Source: CAD feature listing. Evaluate the final solid. Frame: model axes, mm. A direction names the side the tool comes from. Coordinates: 2 decimals unless noted, no trailing zeros. Order: outer loops, then holes, each group sorted by start corner. A loop starts at its lowest first (then second) coordinate and runs counter-clockwise, first axis right, second up. Notation, with made-up numbers: (-37.5, -12.75) -> (-22.5, -12.75) arc R12 ccw to (-22.5, 2.25) -> close; hole circle Ø6 at (-4, 84.5). An arc over 180 degrees is marked (long way). Put each result on its own line as item: value.
from build123d import *

# Parameters (mm, degrees)
F1_DEPTH = 1200
F2_R     = 2


# Not quite as in the source:
# - a feature names something its author has since deleted; it is built from what else it names


with BuildPart() as f1:
    # F0 (on Right) → F1 (new body)
    with BuildSketch(Plane.YZ):
        Polygon((-19.8378913403, 177.8021101952), (-19.8378913403, 154.8021101952), (-17.8378913403, 154.8021101952), (-17.8378913403, 179.8021101952), (-57.8378913403, 179.8021101952), (-57.8378913403, 79.8021101952), (-29.8378913403, 79.8021101952), (-29.8378913403, 53.8021101952), (-27.8378913403, 53.8021101952), (-27.8378913403, 81.8021101952), (-55.8378913403, 81.8021101952), (-55.8378913403, 177.8021101952), align=None)
    extrude(amount=F1_DEPTH)

    # F2
    f2_edges = [f1.edges().sort_by_distance(p)[0] for p in [
        (600, -57.837891, 179.80211),
        (600, -17.837891, 179.80211),
        (600, -57.837891, 79.80211),
        (600, -27.837891, 81.80211),
        (600, -55.837891, 81.80211),
        (600, -29.837891, 79.80211),
        (600, -19.837891, 177.80211),
        (600, -55.837891, 177.80211),
    ]]
    fillet(f2_edges, radius=F2_R)


solid = f1.part
1. Set-up query: faces 5 (the flat face through (1200, -57, 126)), 6 (the flat face through (592, -55.838, 129)), 7 (the flat face through (592, -17.838, 166)), 8 (the flat face through (592, -29.838, 66)), 9 (the flat face through (592, -19.838, 165)). Return all of +Z, -Z, +X, -X, +Y, -Y with unobstructed straight access to the full face (end or side cutting, diameter ignored); none if empty.
Numbers:
face 5: +Z, -Z, +X, +Y, -Y
face 6: +X, -X
face 7: +Z, -Z, +X, -X, +Y
face 8: -Z, +X, -X, -Y
face 9: -Z, +X, -X
2. First-contact query: pin 1 (5 mm diameter, centred on x = 721.5, z = 137.5, fed in from +Y); pin 2 (1 mm diameter, centred on x = 772.5, y = -27, fed in from -Z); pin 3 (9.5 mm diameter, centred on x = 785, y = -38, fed in from -Z). Flat tips, straight axial feed; report the tip coordinate or a pass-through.
Numbers:
pin 1: stops at y = -55.84
pin 2: stops at z = 177.8
pin 3: stops at z = 79.8
3. Ray query, line 1 along Z through (x, y) = (892, -32); line 2 along Y through (x, z) = (1001.5, 172); line 3 along Z through (x, y) = (277, -24.5). Return the intervals inside material, ascending.
Numbers:
line 1: z = 79.8 to 81.8, 177.8 to 179.8
line 2: y = -57.84 to -55.84, -19.84 to -17.84
line 3: z = 177.8 to 179.8
4. Cut plane A-A on y = -47.5. Output: boundary loops of the cut face in (x, z), plus the area to 3 significant figures.
Numbers:
outline: (0, 79.8) -> (1200, 79.8) -> (1200, 81.8) -> (0, 81.8) -> close; (0, 177.8) -> (1200, 177.8) -> (1200, 179.8) -> (0, 179.8) -> close
area: 4,800 mm2
5. Cut plane C-C on z = 110.5. Output: boundary loops of the cut face in (x, y).
Numbers:
outline: (0, -57.84) -> (1200, -57.84) -> (1200, -55.84) -> (0, -55.84) -> close
6. Pull-direction query (Z, two-part tool) for faces 1 (the flat face through (592, -38, 179.802)), 2 (the flat face through (592, -42, 81.802)), 3 (the flat face through (592, -27.838, 67)), 4 (the flat face through (592, -38, 177.802)); classes: pulls with the +Z half, pulls with the -Z half, needs draft (parallel to the pull), parting line crosses it, or undercut.
Numbers:
face 1: pulls with the +Z half
face 2: undercut
face 3: needs draft
face 4: undercut
7. Cut plane B-B on x = 1115. Output: boundary loops of the cut face in (y, z), plus the area to 3 significant figures.
Numbers:
outline: (-57.84, 81.8) arc R2 ccw to (-55.84, 79.8) -> (-31.84, 79.8) arc R2 cw to (-29.84, 77.8) -> (-29.84, 53.8) -> (-27.84, 53.8) -> (-27.84, 79.8) arc R2 ccw to (-29.84, 81.8) -> (-53.84, 81.8) arc R2 cw to (-55.84, 83.8) -> (-55.84, 175.8) arc R2 cw to (-53.84, 177.8) -> (-21.84, 177.8) arc R2 cw to (-19.84, 175.8) -> (-19.84, 154.8) -> (-17.84, 154.8) -> (-17.84, 177.8) arc R2 ccw to (-19.84, 179.8) -> (-55.84, 179.8) arc R2 ccw to (-57.84, 177.8) -> close
area: 430 mm2
